Read the model definition and answer for the solid it produces. Units are mm, in the model's axes. Face numbers are marked on the shaded views. A direction names the side the tool comes from. Give positions to 0.01 mm unless a question says otherwise; leave off trailing zeros. Order: outer loops, then holes, each group sorted by start corner. A loop starts at its lowest first (then second) coordinate and runs counter-clockwise, first axis right, second up. Notation, with made-up numbers: (-25.5, 19.25) - (9.5, 19.25) arc R27 ccw to (9.5, 46.25) - close; hole circle Ø3 at (24.25, 39). An arc over 180 degrees is marked (long way). Write each question's results on one line, items separated by ' | '.
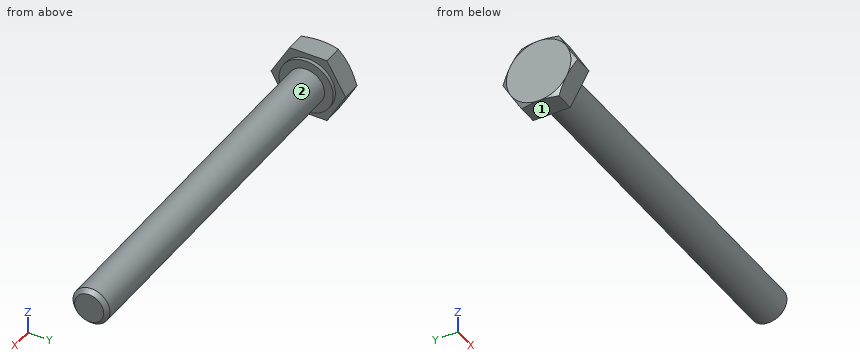
Autodesk Inventor part; units mm, degrees
ref_plane "Work Plane1" through (1.525, 0, 0) normal (0, 0, 1) x (1, 0, 0)
ref_plane "YZ Plane" through (0, 0, 0) normal (1, 0, 0) x (0, 1, 0)
ref_plane "XZ Plane" through (0, 0, 0) normal (0, 1, 0) x (-1, 0, 0)
sketch "Sketch1" plane through (0, 0, 0) normal (0, 0, 1) x (1, 0, 0)
  line L0 (0, 2.94) -> (0, 2)
  line L1 (2.1, 2) -> (40, 2)
  line L2 (40, 2) -> (40, 0)
  line L3 (40, 0) -> (-0.4001, 0)
  line L4 (-8.4801, 0) -> (48.08, 0)
  line L5 (-0.4001, 0) -> (-0.4001, 2.94)
  line L6 (-0.4001, 2.94) -> (0, 2.94)
  line L7 (2.1, 2) -> (1.6705, 2)
  line L8 (1.6705, 2) -> (0, 2)
  line L9 (0, -0.588) -> (0, 3.528)
  dimension "d0" = 40
  dimension "d1" = 37.9
  dimension "d2" = 4
  dimension "d9" = 0.4001
  dimension "d10" = 5.88
  dimension "d13" = 0.4295
  dimension "d14" = 4
revolve "Body" add sketch "Sketch1" angle 360 about axis through (40, 0, 0) along (-1, 0, 0)
sketch "Sketch2" plane through (-0.4001, 0, 0) normal (-1, 0, 0) x (0, 0, 1)
  line L0 (0, 4.0415) -> (3.5, 2.0207)
  line L1 (3.5, 2.0207) -> (3.5, -2.0207)
  line L2 (3.5, -2.0207) -> (0, -4.0415)
  line L3 (0, -4.0415) -> (-3.5, -2.0207)
  line L4 (-3.5, -2.0207) -> (-3.5, 2.0207)
  line L5 (-3.5, 2.0207) -> (0, 4.0415)
  point P0 (0, 0)
  point P1 (0, 0)
  dimension "d11" = 7
extrude "Head" add sketch "Sketch2" along normal blind 2.4
sketch "Sketch4" plane through (0, 0, 0) normal (0, 0, 1) x (1, 0, 0)
  line L0 (-2.8001, 3.5) -> (-2.8001, 4.0415)
  line L1 (-2.8001, 4.0415) -> (-2.4875, 4.0415)
  line L2 (-2.4875, 4.0415) -> (-2.8001, 3.5)
  line L3 (-3.2801, 0) -> (0.0799, 0)
  line L4 (-0.4001, 4.0415) -> (-2.8001, 4.0415)
  line L5 (-2.8001, 2.0207) -> (-2.8001, 4.0415)
  dimension "d5" = 30
  dimension "d19" = 7
revolve "Chamfer1" cut sketch "Sketch4" angle 360 about axis through (-10, 0, 0) along (1, 0, 0)
thread "Thread"
chamfer "Chamfer2" distance 0.4294 distance2 0.4295 1 edges at (40, -2, 0) measured on face at (40, -0.499, -0.4421)
ref_plane "Work Plane1" through (1.525, 0, 0) normal (0, 0, 1) x (1, 0, 0)
equation "\"d0\" = NLG"
equation "\"d1\" = GEL"
equation "\"d2\" = GD"
equation "\"d10\" = SD2"
equation "\"d14\" = BDM"
equation "\"d11\" = SW"
equation "\"d3\" = KOH - SD"
equation "\"d5\" = ANG1"
equation "\"d19\" = SW0"
equation "\"d15\" = GEL"
equation "\"d6\" = -0.5 * SPD + 0.5 * GD"
equation "\"NLG\" = 40"
equation "\"GD\" = NND"
equation "\"BDM\" = NND"
equation "\"KOH\" = 2.8"
equation "\"GEL\" = 37.9"
equation "\"SW\" = 7"
equation "\"SW0\" = SW"
equation "\"SPD\" = NND - 1.2269 * PTC"
equation "\"SD2\" = 5.88"
equation "\"SD\" = 0.4"
equation "\"ANG1\" = 30deg"
equation "\"GAL\" = 0.61345 * PTC"
equation "\"GUL\" = 0.61345 * PTC"
equation "\"RR\" = 0.2"
equation "\"GD1\" = THREADDIA - 1.2269 * PTC"
equation "\"THREADDIA\" = 4"
equation "\"SDH\" = SD2"
equation "\"SDHG\" = 2.1"
equation "\"TOA\" = 30deg"
equation "\"PTC\" = 0.7"
equation "\"NND\" = 4"
equation "\"E0\" = 8.085"
properties part number "ISO 4017 - M4 x 40(3)" material "Stainless Steel, 440C"
(1) Each of these flat-tipped pins is pushed along its axis until it touches: pin 1 (3 mm diameter, centred on x = 32, z = 0, fed in from -Y); pin 2 (1 mm diameter, centred on x = 31, z = -2, fed in from +Y); pin 3 (2 mm diameter, centred on x = 7, z = 0.5, fed in from +Y). Where does it stop, or does it pass through?
Conclusion:
pin 1: y = -2 | pin 2: y = 1.32 | pin 3: y = 2
(2) Consider probe 1 along Z at (x, y) = (26, 0); probe 2 along Z at (x, y) = (17, 1.25); probe 3 along X at (y, z) = (-2.5, -0.5). Determine where each line is inside the solid, lowest interval first. Write a range as [from, to].
Conclusion:
probe 1: [-2, 2] | probe 2: [-1.56, 1.56] | probe 3: [-2.8, 0]
(3) For the marked faces 1 and 2, determine the directions among +Z, -Z, +X, -X, +Y, -Y from which every point of the face is accessible in a straight line to the end or side of a thin tool.
Conclusion:
face 1: -Z, +X, -X, +Y, -Y | face 2: +X
(4) Section A-A (x = 0.5) is taken. Give the vertices of the cut face in (y, z), plus the area to 3 significant figures.
Conclusion:
outline: circle Ø4 at (0, 0) | area: 12.6 mm^2
